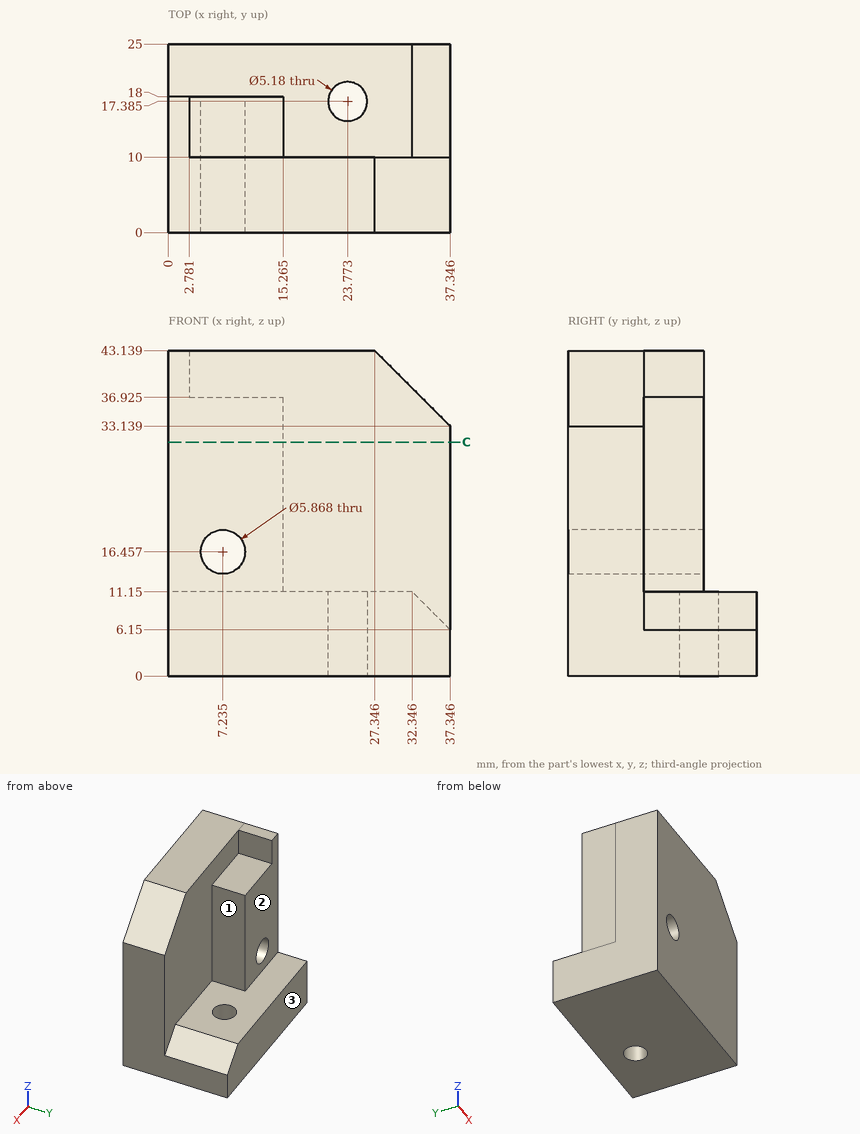
Answer from the drawing. Dimensions are ordinates in mm from the lowest x, y and z of the part. A direction names the side the tool comes from. Give positions to 0.01 mm unless a question says otherwise; leave off trailing zeros. Write each loop counter-clockwise with the first axis right and the second up, starting at its lowest first coordinate (ties: lowest second). Pieces come first, ordered by that corner, then holes. Notation, with made-up numbers: (-38, 54) -> (-28, 54) arc R18 cw to (-28, 80) -> close; hole circle Ø4 at (-31.75, 89.5). An arc over 180 degrees is marked (long way). Use a Markdown table: item, result.
(1) Section C-C, the plane z = 31 is taken. Determine the outline of the cut face in (x, y) (1 decimal).
Return value:
| item | result |
|---|---|
| outline | (0, 0) -> (37.3, 0) -> (37.3, 10) -> (15.3, 10) -> (15.3, 18) -> (0, 18) -> close |
(2) Find the intervals of material crossed by probe 1 along Y at (x, z) = (18, 39); probe 2 along X at (y, z) = (6, 17.5) (1 decimal); probe 3 along Z at (x, y) = (27.5, 22), in increasing order. Write a range as from..to.
Return value:
| item | result |
|---|---|
| probe 1 | 0..10 |
| probe 2 | 0..4.5, 10..37.3 |
| probe 3 | 0..11.15 |
(3) Flat-ended cylindrical pins translate along their axes: P1, Ø5, axis at y = 16, z = 40.5, coming from the +X side; P2, Ø12, axis at x = 20, z = 25.5, coming from the +Y side; P3, Ø10, axis at x = 24, z = 28.5, coming from the +Y side. Find the tip coordinate at first contact, or state that the pin passes through.
Return value:
| item | result |
|---|---|
| P1 | x = 2.78 |
| P2 | y = 18 |
| P3 | y = 10 |
(4) For the marked faces 1, 2 and 3, determine the directions among +Z, -Z, +X, -X, +Y, -Y from which every point of the face is accessible in a straight line to the end or side of a thin tool.
Return value:
| item | result |
|---|---|
| face 1 | +Z, +X, +Y |
| face 2 | +Z, +X, -X, +Y |
| face 3 | +Z, -Z, +X, -X, +Y |
